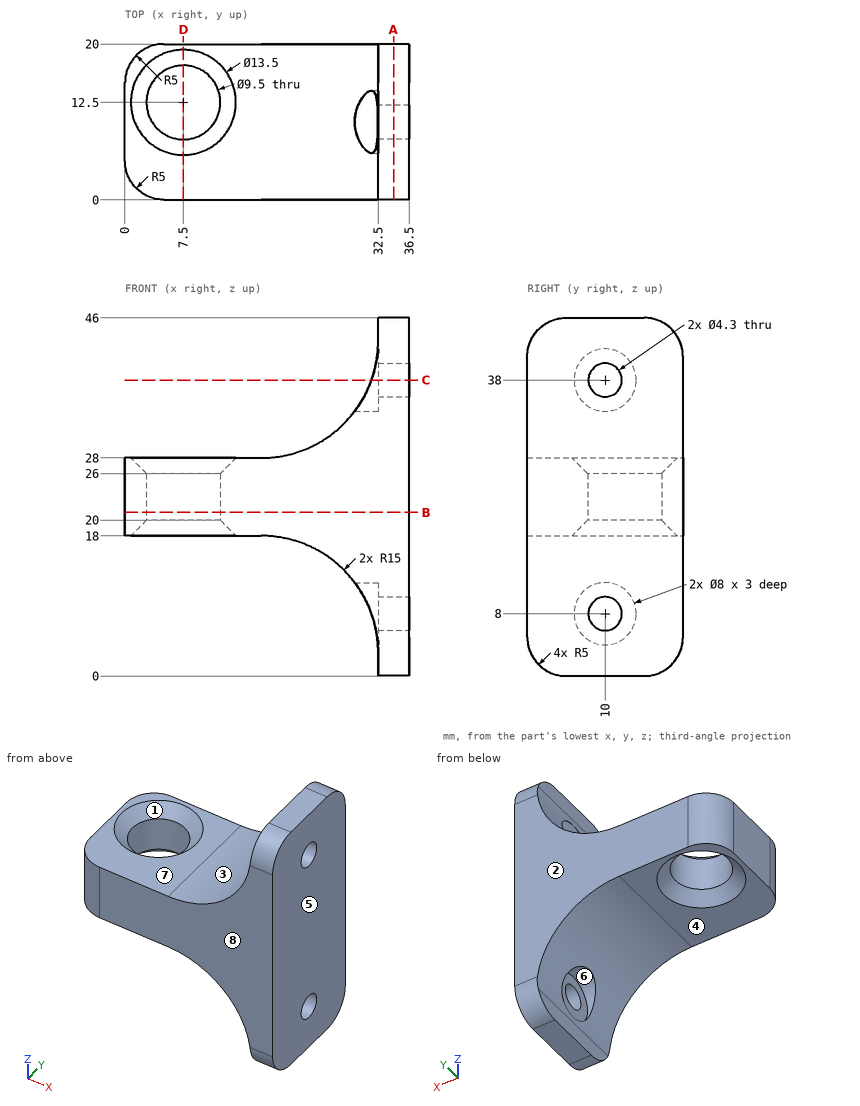
Answer from the drawing. Dimensions are ordinates in mm from the lowest x, y and z of the part. A direction names the side the tool comes from. Give positions to 0.01 mm unless a question says otherwise; leave off trailing zeros. Order: outer loops, then holes, each group sorted by start corner. A loop starts at its lowest first (then second) coordinate and runs counter-clockwise, first axis right, second up.
Item 1: Find the intervals of material crossed by probe 1 along Z at (x, y) = (34.2, 10); probe 2 along X at (y, z) = (14.75, 41); probe 3 along Z at (x, y) = (30.4, 10), in increasing order.
From the geometry:
probe 1: z = 0 to 5.85, 10.15 to 35.85, 40.15 to 46
probe 2: x = 32.37 to 36.5
probe 3: z = 12 to 34
Item 2: For a pull along X with two mould halves and no side action, classify the marked faces 1, 2 and 3 as pulls with the +X half, pulls with the -X half, needs draft (parallel to the pull), parting line crosses it, or undercut.
From the geometry:
face 1: undercut
face 2: needs draft
face 3: pulls with the -X half
Item 3: The part is cut by section A-A, the plane x = 34.5. Give the vertices of the cut face in (y, z), and give its area (3 significant figures).
From the geometry:
outline: (0, 5) arc R5 ccw to (5, 0) - (15, 0) arc R5 ccw to (20, 5) - (20, 41) arc R5 ccw to (15, 46) - (5, 46) arc R5 ccw to (0, 41) - close; hole circle Ø4.3 at (10, 8); hole circle Ø4.3 at (10, 38)
area: 869 mm2
Item 4: The part is cut by section C-C, the plane z = 38. Give the vertices of the cut face in (x, y).
From the geometry:
outline: (31.64, 0) - (36.5, 0) - (36.5, 7.85) - (32.5, 7.85) - (32.5, 6) - (31.64, 6) - close; (31.64, 14) - (32.5, 14) - (32.5, 12.15) - (36.5, 12.15) - (36.5, 20) - (31.64, 20) - close
Item 5: The part is cut by section D-D, the plane x = 7.5. Give the vertices of the cut face in (y, z), and give its area (3 significant figures).
From the geometry:
outline: (0, 18) - (5.75, 18) - (7.75, 20) - (7.75, 26) - (5.75, 28) - (0, 28) - close; (17.25, 20) - (19.25, 18) - (20, 18) - (20, 28) - (19.25, 28) - (17.25, 26) - close
area: 97.0 mm2
Item 6: Given pin 1 Ø1.5 at (y, z) = (6.5, 8.5) entering from -X; pin 2 Ø1.5 at (x, y) = (29.5, 8.5) entering from -Z; pin 3 Ø2.5 at (y, z) = (8, 7) entering from -X, each flat-ended and moving along its own axis, determine where each tip first touches the part or whether it passes through.
From the geometry:
pin 1: stops at x = 31.17
pin 2: stops at z = 11.4
pin 3: stops at x = 32.5
Item 7: The part is cut by section B-B, the plane z = 21. Give the vertices of the cut face in (x, y), and give its area (3 significant figures).
From the geometry:
outline: (0, 5) arc R5 ccw to (5, 0) - (36.5, 0) - (36.5, 20) - (5, 20) arc R5 ccw to (0, 15) - close; hole circle Ø9.5 at (7.5, 12.5)
area: 648 mm2
Item 8: Which of the six approach directions +Z, -Z, +X, -X, +Y, -Y give full straight-line access (tool end or side, diameter ignored) to the marked faces 4, 5, 6, 7 and 8?
From the geometry:
face 4: -Z, -X, +Y, -Y
face 5: +Z, -Z, +X, +Y, -Y
face 6: -X
face 7: +Z, -X, +Y, -Y
face 8: +Z, -Z, +X, -X, -Y
